Could you check a few things on this model? Use its own coordinates, in mm. A direction names the side the tool comes from. Give positions to 0.01 mm unless a question says otherwise; leave off trailing zeros. Order: outer loops, then holes, each group sorted by start corner. A loop starts at its lowest first (then second) coordinate and runs counter-clockwise, first axis right, second up. Notation, with made-up numbers: (55.5, 53) -> (68.5, 53) arc R15 ccw to (68.5, 79) -> close; hole circle Ø11 at (48.5, 15). An arc over 180 degrees is marked (long way). Use one line per item in the form item = value. Start each with the question number.
from build123d import *

# Parameters (mm, degrees)
SKETCH_R        = 1.7
PAD_DEPTH       = 13
SKETCH001_W     = 82
SKETCH001_H     = 101
POCKET_DEPTH    = 10
SKETCH002_W     = 18.5
SKETCH002_H     = 7.5
POCKET001_DEPTH = 11
SKETCH003_R     = 3
POCKET002_DEPTH = 3.1


with BuildPart() as part:
    # Sketch → Pad (new body)
    with BuildSketch(Plane.XY):
        with BuildLine():
            Line((-5, 0), (-5, -110))
            ThreePointArc((-5, -110), (-3.535534, -113.535534), (0, -115))
            Line((0, -115), (91, -115))
            ThreePointArc((91, -115), (94.535534, -113.535534), (96, -110))
            Line((96, -110), (96, 0))
            ThreePointArc((96, 0), (94.535534, 3.535534), (91, 5))
            Line((91, 5), (0, 5))
            ThreePointArc((0, 5), (-3.535534, 3.535534), (-5, 0))
        make_face()
        Circle(SKETCH_R, mode=Mode.SUBTRACT)
        with Locations((91, 0)):
            Circle(SKETCH_R, mode=Mode.SUBTRACT)
        with Locations((91, -110)):
            Circle(SKETCH_R, mode=Mode.SUBTRACT)
        with Locations((0, -110)):
            Circle(SKETCH_R, mode=Mode.SUBTRACT)
    extrude(amount=PAD_DEPTH)

    # Sketch001 (on Face14 of Pad) → Pocket (cut)
    with BuildSketch(Plane.XY.offset(13)):
        with Locations((45.5, -55)):
            Rectangle(SKETCH001_W, SKETCH001_H)
    extrude(amount=-POCKET_DEPTH, mode=Mode.SUBTRACT)

    # Sketch002 (on Face1 of Pocket) → Pocket001 (cut)
    with BuildSketch(Plane(origin=(-5, 0, 0), x_dir=(0, -1, 0), z_dir=(-1, 0, 0))):
        with Locations((16, 9.25)):
            Rectangle(SKETCH002_W, SKETCH002_H)
    extrude(amount=-POCKET001_DEPTH, mode=Mode.SUBTRACT)

    # Sketch003 (on Face2 of Pocket001) → Pocket002 (cut)
    with BuildSketch(Plane(origin=(0, 0, 0), x_dir=(1, 0, 0), z_dir=(0, 0, -1))):
        with Locations((0, 110)):
            Circle(SKETCH003_R)
        with Locations((91, 110)):
            Circle(SKETCH003_R)
        with Locations((91, 0)):
            Circle(SKETCH003_R)
        Circle(SKETCH003_R)
    extrude(amount=-POCKET002_DEPTH, mode=Mode.SUBTRACT)


solid = part.part
(1) I'm going to push flat-ended pins straight in: pin 1 Ø3 at (x, y) = (-1, -111) entering from -Z; pin 2 Ø9.5 at (x, y) = (0, 0) entering from +Z; pin 3 Ø1 at (x, y) = (52, -35) entering from +Z; pin 4 Ø3 at (x, y) = (2, -17.5) entering from +Z. Where does each tip first touch, or does it pass through?
(2) We'd pull the mould along X, two halves only. Please class faces 6 (the flat face through (0, -25.25, 9)), 7 (the flat face through (-5, -54, 6)), 8 (the flat face through (91, -108, 3.1)), 9 (the cylindrical face through (-2.4, -108.2, 1.5)): pulls with the +X half, pulls with the -X half, needs draft (parallel to the pull), parting line crosses it, or undercut.
(3) Imagine slicing it at A-A (z = 9.5). Write out the boundary of the cut face in (x, y), plus the area to 3 significant figures.
(4) Which directions (+Z, -Z, +X, -X, +Y, -Y) give clear straight access to the entire face, cutting with the end or side of a thin tool? Please do faces 1 (the flat face through (45, -115, 6)), 2 (the flat face through (2, -110, 3.1)), 3 (the cylindrical face through (94, -114, 6)), 4 (the flat face through (0, -16, 5.5)), 5 (the flat face through (86.5, -56, 8)).
(5) Imagine slicing it at B-B (y = -12). Write out the boundary of the cut face in (x, z).
(6) Please list where these lines run through material, in increasing order: probe 1 along Y at (x, z) = (91, 1.05); probe 2 along Y at (x, z) = (91, 11); probe 3 along X at (y, z) = (-110, 2.2).
(7) Imagine slicing it at C-C (x = 53.5). Write out the boundary of the cut face in (y, z).
Calculated:
q1.pin_1 = 3.1
q1.pin_2 = 13
q1.pin_3 = 3
q1.pin_4 = 5.5
q2.face_6 = needs draft
q2.face_7 = pulls with the -X half
q2.face_8 = undercut
q2.face_9 = undercut
q3.outline = (-5, -110) arc R5 ccw to (0, -115) -> (91, -115) arc R5 ccw to (96, -110) -> (96, 0) arc R5 ccw to (91, 5) -> (0, 5) arc R5 ccw to (-5, 0) -> (-5, -6.75) -> (4.5, -6.75) -> (4.5, -4.5) -> (86.5, -4.5) -> (86.5, -105.5) -> (4.5, -105.5) -> (4.5, -25.25) -> (-5, -25.25) -> close; hole circle Ø3.4 at (0, -110); hole circle Ø3.4 at (0, 0); hole circle Ø3.4 at (91, -110); hole circle Ø3.4 at (91, 0)
q3.area = 3,600 mm2
q4.face_1 = +Z, -Z, +X, -X, -Y
q4.face_2 = -Z
q4.face_3 = +Z, -Z, +X, -Y
q4.face_4 = +Z, -X
q4.face_5 = +Z
q5.outline = (-5, 0) -> (96, 0) -> (96, 13) -> (86.5, 13) -> (86.5, 3) -> (4.5, 3) -> (4.5, 5.5) -> (-5, 5.5) -> close
q6.probe_1 = -115 to -113, -107 to -3, 3 to 5
q6.probe_2 = -115 to -111.7, -108.3 to -1.7, 1.7 to 5
q6.probe_3 = -5 to -3, 3 to 88, 94 to 96
q7.outline = (-115, 0) -> (5, 0) -> (5, 13) -> (-4.5, 13) -> (-4.5, 3) -> (-105.5, 3) -> (-105.5, 13) -> (-115, 13) -> close
